Source: CAD feature listing. Evaluate the final solid. Frame: model axes, mm. Face numbers are marked on the shaded views. A direction names the side the tool comes from. Give positions to 0.01 mm unless a question says otherwise; leave off trailing zeros. Order: outer loops, then holes, each group sorted by start corner. A loop starts at its lowest first (then second) coordinate and runs counter-clockwise, first axis right, second up. Notation, with made-up numbers: M 72,-34.75 L 116,-34.75 A31 cw 116,-5.75 Z; hole C 17,-2 d8. An arc over 180 degrees is marked long. Use CSV: the item, a comma, the result in double quotes. Start each with the question number.
Item 1: Pull-direction query (X, two-part tool) for the marked faces 1, 2, 3 and 4; classes: +X half, -X half, draft (parallel to the pull), parting line (faces both ways), or undercut.
Item 2: Section query B-B on z = 8.5. Return loops of the section in (x, y), and give its area (3 significant figures).
Item 3: Section query D-D on z = 19. Return loops of the section in (x, y).
Item 4: Access query for the marked faces 5, 6, 7, 8 and 9. Directions: +Z, -Z, +X, -X, +Y, -Y. A direction counts if a zero-diameter tool reaches every point of the face in a straight line with its end or side. Return the directions, or none.
Item 5: First-contact query: pin 1 (5 mm diameter, centred on x = 12.5, z = 20, fed in from -Y); pin 2 (1.5 mm diameter, centred on x = 19.5, y = 24, fed in from +Z); pin 3 (1 mm diameter, centred on x = 18, z = 5.5, fed in from +Y). Flat tips, straight axial feed; report the tip coordinate or a pass-through.
Item 6: Section query C-C on x = 13. Count the separate pieces of the cut face and the enclosed holes in it, and give its area (3 significant figures).
Item 7: Section query A-A on y = 9. Return loops of the section in (x, z).
Item 8: Ray query, probe 1 along X at (y, z) = (21.3, 20); probe 2 along Y at (x, z) = (12.5, 4.25); probe 3 along Y at (x, z) = (12.5, -14.5). Return the intervals inside material, ascending. Write a range as from..to.
from build123d import *

# Parameters (mm, degrees)
SKETCH1_R           = 2.65
BOSS_EXTRUDE1_DEPTH = 10
BOSS_EXTRUDE2_START = -20
SKETCH2_W           = 25
SKETCH2_H           = 20
BOSS_EXTRUDE2_DEPTH = 5
BOSS_EXTRUDE3_DEPTH = 5
SKETCH4_W           = 25
SKETCH4_H           = 7.5
BOSS_EXTRUDE4_DEPTH = 20
SKETCH5_W           = 10
SKETCH5_H           = 20
BOSS_EXTRUDE5_DEPTH = 8
FILLET2_R           = 2
SKETCH6_R           = 2.75
CUT_EXTRUDE1_DEPTH  = 6
SKETCH7_R           = 2.75
CUT_EXTRUDE2_DEPTH  = 6
BOSS_EXTRUDE6_START = -8
BOSS_EXTRUDE6_DEPTH = 8
SKETCH9_R           = 2.65
CUT_EXTRUDE3_DEPTH  = 50
FILLET4_R           = 2
FILLET6_R           = 2


with BuildPart() as part:
    # Sketch1 → Boss-Extrude1 (new body)
    with BuildSketch(Plane.XY):
        with BuildLine():
            Line((0, 0), (25, 0))
            Line((25, 0), (25, 40))
            ThreePointArc((25, 40), (22.071067812, 47.071067812), (15, 50))
            Line((15, 50), (10, 50))
            ThreePointArc((10, 50), (2.928932188, 47.071067812), (0, 40))
            Line((0, 40), (0, 0))
        make_face()
        with Locations((12.5, 35)):
            Circle(SKETCH1_R, mode=Mode.SUBTRACT)
    extrude(amount=BOSS_EXTRUDE1_DEPTH)

    # Sketch2 → Boss-Extrude2 (add)
    with BuildSketch(Plane.XZ.offset(BOSS_EXTRUDE2_START)):
        with Locations((12.5, 20)):
            Rectangle(SKETCH2_W, SKETCH2_H)
    extrude(amount=-BOSS_EXTRUDE2_DEPTH)

    # Sketch3 → Boss-Extrude3 (add)
    with BuildSketch(Plane.XZ):
        Polygon((0, 0), (25, 0), (25, 10), (25, 30), (0, 30), (0, 10), align=None)
    extrude(amount=BOSS_EXTRUDE3_DEPTH)

    # Sketch4 → Boss-Extrude4 (add)
    with BuildSketch(Plane(origin=(0, 0, 0), x_dir=(-1, 0, 0), z_dir=(0, 0, -1))):
        with Locations((-12.5, -1.25)):
            Rectangle(SKETCH4_W, SKETCH4_H)
    extrude(amount=BOSS_EXTRUDE4_DEPTH)

    # Sketch5 → Boss-Extrude5 (add)
    with BuildSketch(Plane(origin=(0, 0, -20), x_dir=(-1, 0, 0), z_dir=(0, 0, -1))):
        with Locations((-12.5, 12.5)):
            Rectangle(SKETCH5_W, SKETCH5_H)
    extrude(amount=-BOSS_EXTRUDE5_DEPTH)

    # Fillet2
    fillet2_edges = [part.edges().sort_by_distance(p)[0] for p in [
        (12.5, 2.5, 0),
        (12.5, 2.5, -12),
    ]]
    fillet(fillet2_edges, radius=FILLET2_R)

    # Sketch6 → Cut-Extrude1 (cut)
    with BuildSketch(Plane(origin=(0, 25, 0), x_dir=(1, 0, 0), z_dir=(0, 1, 0))):
        with Locations((5, -20)):
            Circle(SKETCH6_R)
        with Locations((20, -20)):
            Circle(SKETCH6_R)
    extrude(amount=-CUT_EXTRUDE1_DEPTH, mode=Mode.SUBTRACT)

    # Sketch7 → Cut-Extrude2 (cut)
    with BuildSketch(Plane.XZ.offset(5)):
        with Locations((12.5, 20)):
            Circle(SKETCH7_R)
    extrude(amount=-CUT_EXTRUDE2_DEPTH, mode=Mode.SUBTRACT)

    # Sketch8 → Boss-Extrude6 (add)
    with BuildSketch(Plane(origin=(0, 0, -20), x_dir=(-1, 0, 0), z_dir=(0, 0, -1)).offset(BOSS_EXTRUDE6_START)):
        with BuildLine():
            Line((-17.5, 22.5), (-17.5, 35))
            ThreePointArc((-17.5, 35), (-12.5, 40), (-7.5, 35))
            Line((-7.5, 35), (-7.5, 22.5))
            Line((-7.5, 22.5), (-17.5, 22.5))
        make_face()
    extrude(amount=BOSS_EXTRUDE6_DEPTH)

    # Sketch9 → Cut-Extrude3 (cut)
    with BuildSketch(Plane(origin=(0, 0, -20), x_dir=(-1, 0, 0), z_dir=(0, 0, -1))):
        with Locations((-12.5, 35)):
            Circle(SKETCH9_R)
    extrude(amount=-CUT_EXTRUDE3_DEPTH, mode=Mode.SUBTRACT)

    # Fillet4
    fillet4_edges = [part.edges().sort_by_distance(p)[0] for p in [
        (12.5, 25, 10),
    ]]
    fillet(fillet4_edges, radius=FILLET4_R)

    # Fillet6
    fillet6_edges = [part.edges().sort_by_distance(p)[0] for p in [
        (12.5, 25, 30),
        (0, 22.5, 30),
        (25, 22.5, 30),
        (25, -2.5, 30),
        (0, -2.5, 30),
        (12.5, -5, 30),
    ]]
    fillet(fillet6_edges, radius=FILLET6_R)


solid = part.part
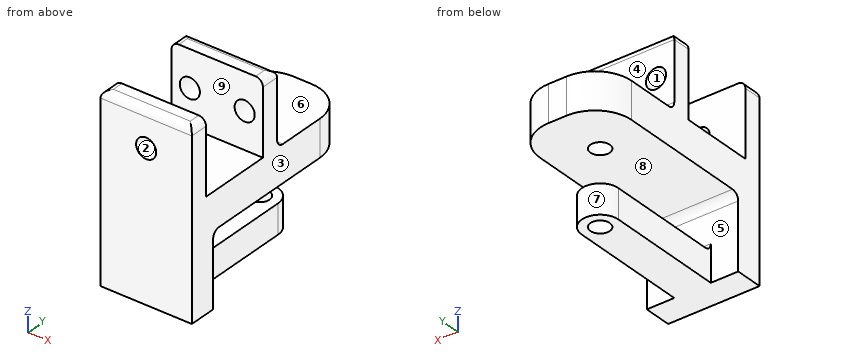
Verdict:
1,face 1,"undercut"
1,face 2,"undercut"
1,face 3,"+X half"
1,face 4,"draft"
2,outline,"M 0,-5 L 25,-5 L 25,40 A10 ccw 15,50 L 10,50 A10 ccw 0,40 Z; hole C 12.5,35 d5.3"
2,area,"1,310 mm2"
3,outline,"M 0,-5 L 9.94,-5 L 9.94,0 L 0,0 Z; M 0,20 L 2.44,20 L 2.44,25 L 0,25 Z; M 7.56,20 L 17.44,20 L 17.44,25 L 7.56,25 Z; M 15.06,-5 L 25,-5 L 25,0 L 15.06,0 Z; M 22.56,20 L 25,20 L 25,25 L 22.56,25 Z"
4,face 5,"+Y"
4,face 6,"+Z, +X, -X, +Y"
4,face 7,"-Z, +Y"
4,face 8,"+X, -X, +Y"
4,face 9,"+Z, +X, -X"
5,pin 1,"y = 20"
5,pin 2,"z = 29.98"
5,pin 3,"y = 49.68"
6,separate pieces,"4"
6,enclosed holes,"0"
6,area,"1,080 mm2"
7,outline,"M 0,0 L 25,0 L 25,10 L 0,10 Z; M 7.5,-20 L 17.5,-20 L 17.5,-12 L 7.5,-12 Z"
8,probe 1,"0..2.25, 7.75..17.25, 22.75..25"
8,probe 2,"-5..32.35, 37.65..50"
8,probe 3,"-5..32.35, 37.65..40"
